from build123d import *

# Parameters (mm, degrees)
F1_DEPTH  = 25.4
F3_DEPTH  = 25.4
F5_DEPTH  = 25.4
F7_DEPTH  = 25.4
F8_R      = 5.661864
F8_R_2    = 5.740655
F9_DEPTH  = 25.4
F10_R     = 6.51074
F11_DEPTH = 25.4


with BuildPart() as f1:
    # F0 (on Front) → F1 (new body)
    with BuildSketch(Plane.XZ):
        Polygon((-57.679164, 12.697244), (-57.414579, 0), (18.520836, 0), (18.520836, 12.697244), (-6.879164, 12.697244), (-6.879164, 32.676041), (-32.279164, 32.676041), (-32.279164, 12.697244), align=None)
    extrude(amount=F1_DEPTH)

    # F2 (on face) → F3 (cut)
    with BuildSketch(Plane.YZ.offset(-6.879164)):
        with BuildLine():
            ThreePointArc((-25.4, 22.686642), (-21.850641, 29.175992), (-15.334563, 32.676041))
            Line((-15.334563, 32.676041), (-25.4, 32.676041))
            Line((-25.4, 32.676041), (-25.4, 22.686642))
        make_face()
        with BuildLine():
            ThreePointArc((-10.065437, 32.676041), (-3.549359, 29.175992), (0, 22.686642))
            Line((0, 22.686642), (0, 32.676041))
            Line((0, 32.676041), (-10.065437, 32.676041))
        make_face()
    extrude(amount=-F3_DEPTH, mode=Mode.SUBTRACT)

    # F4 (on face) → F5 (cut)
    with BuildSketch(Plane.XY.offset(12.697244)):
        with BuildLine():
            ThreePointArc((-57.679164, -11.891091), (-55.299332, -4.965624), (-49.917113, 0))
            Line((-49.917113, 0), (-57.679164, 0))
            Line((-57.679164, 0), (-57.679164, -11.891091))
        make_face()
        with BuildLine():
            ThreePointArc((-51.343318, -25.4), (-55.737963, -20.601527), (-57.679164, -14.391054))
            Line((-57.679164, -14.391054), (-57.679164, -25.4))
            Line((-57.679164, -25.4), (-51.343318, -25.4))
        make_face()
    extrude(amount=-F5_DEPTH, mode=Mode.SUBTRACT)

    # F6 (on face) → F7 (cut)
    with BuildSketch(Plane.XY.offset(12.697244)):
        with BuildLine():
            ThreePointArc((8.271978, 0), (18.290982, -12.275574), (9.412941, -25.4))
            Line((9.412941, -25.4), (18.520836, -25.4))
            Line((18.520836, -25.4), (18.520836, 0))
            Line((18.520836, 0), (8.271978, 0))
        make_face()
    extrude(amount=-F7_DEPTH, mode=Mode.SUBTRACT)

    # F8 (on face) → F9 (cut)
    with BuildSketch(Plane.XY.offset(12.697244)):
        with Locations((3.137648, -13.54893)):
            Circle(F8_R)
        with Locations((-42.774935, -13.141072)):
            Circle(F8_R_2)
    extrude(amount=-F9_DEPTH, mode=Mode.SUBTRACT)

    # F10 (on face) → F11 (cut)
    with BuildSketch(Plane.YZ.offset(-6.879164)):
        with Locations((-12.550588, 24.388077)):
            Circle(F10_R)
    extrude(amount=-F11_DEPTH, mode=Mode.SUBTRACT)


solid = f1.part
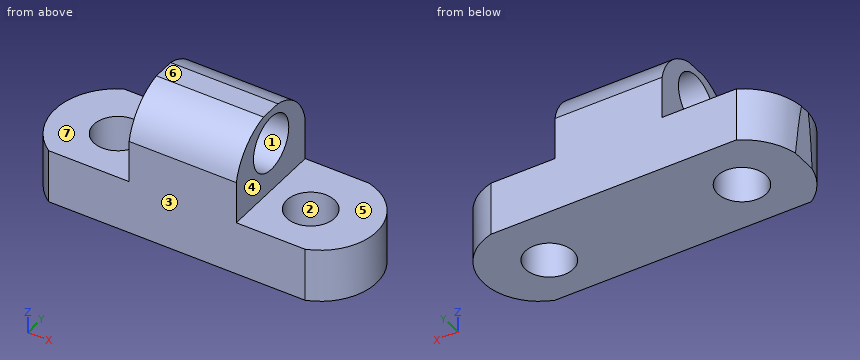
Model file for the job. Use its own axes, mm. Face numbers are marked on the shaded views. A direction names the side the tool comes from. Give positions to 0.01 mm unless a question says otherwise; leave off trailing zeros. Write each loop counter-clockwise with the first axis right and the second up, starting at its lowest first coordinate (ties: lowest second). Pieces come first, ordered by that corner, then holes. Notation, with made-up numbers: (-24.75, 71) -> (28.25, 71) arc R4 ccw to (28.25, 78) -> close; hole circle Ø5 at (71, 27). An arc over 180 degrees is marked (long way). Write item = value, one per line.
(1) Slice it at D-D, the plane x = -21. Give the cut face in (y, z).
Determined:
outline = (-25.4, 0) -> (0, 0) -> (0, 22.69) arc R12.99 ccw to (-10.07, 32.68) -> (-15.33, 32.68) arc R12.99 ccw to (-25.4, 22.69) -> close; hole circle Ø13.02 at (-12.55, 24.39)
(2) Flat gauge pins, fed straight in: P1, Ø12, axis at y = -11, z = 5, coming from the +X side; P2, Ø5, axis at y = -7.5, z = 12.5, coming from the +X side; P3, Ø10, axis at y = -16.5, z = 18.5, coming from the -X side; P4, Ø4, axis at x = 5, z = 15, coming from the +Y side. Where does each tip first touch, or does it go through?
Determined:
P1 = 18.3
P2 = 17.99
P3 = -32.28
P4 = through
(3) Slice it at C-C, the plane y = -11. Give the cut face in (x, z), then the cut area to 3 significant figures.
Determined:
outline = (-57.58, 7.82) -> (-57.41, 0) -> (-48.1, 0) -> (-48.1, 12.7) -> (-57.58, 12.7) -> close; (-37.45, 0) -> (-1.92, 0) -> (-1.92, 12.7) -> (-6.88, 12.7) -> (-6.88, 18.06) -> (-32.28, 18.06) -> (-32.28, 12.7) -> (-37.45, 12.7) -> close; (-32.28, 30.71) -> (-6.88, 30.71) -> (-6.88, 32.68) -> (-32.28, 32.68) -> close; (8.19, 0) -> (18.17, 0) -> (18.17, 12.7) -> (8.19, 12.7) -> close
area = 884 mm2
(4) Probe line 1 along Z through (x, y) = (-40, -7.5); line 2 along Z through (x, y) = (-20.5, -7); line 3 along X through (y, z) = (-16.5, 2). List the from-to ranges inside material, lowest first.
Determined:
line_1 = 0 to 12.7
line_2 = 0 to 20.99, 27.79 to 31.63
line_3 = -57.35 to -47.43, -38.12 to -1.69, 7.97 to 17.8
(5) Mould opens along Y. For the marked faces 1, 2, 3 and 4 say: released by +Y, released by -Y, zero draft, split by the parting line, or undercut.
Determined:
face_1 = undercut
face_2 = undercut
face_3 = released by -Y
face_4 = zero draft
(6) Slice it at A-A, the plane z = 29.5. Give the cut face in (x, y), then the cut area to 3 significant figures.
Determined:
outline = (-32.28, -21.51) -> (-6.88, -21.51) -> (-6.88, -16.58) -> (-32.28, -16.58) -> close; (-32.28, -8.52) -> (-6.88, -8.52) -> (-6.88, -3.89) -> (-32.28, -3.89) -> close
area = 243 mm2
(7) Tool access for the marked faces 5, 6 and 7: list every direction of +Z, -Z, +X, -X, +Y, -Y with a clear straight run to the whole face (end or side of a thin tool).
Determined:
face_5 = +Z, +X, +Y, -Y
face_6 = +Z, +X, -X, +Y, -Y
face_7 = +Z, -X, +Y, -Y
(8) Slice it at B-B, the plane x = -47.5. Give the cut face in (y, z), then the cut area to 3 significant figures.
Determined:
outline = (-25.4, 0) -> (-16.4, 0) -> (-16.4, 12.7) -> (-25.4, 12.7) -> close; (-9.88, 0) -> (0, 0) -> (0, 12.7) -> (-9.88, 12.7) -> close
area = 240 mm2
